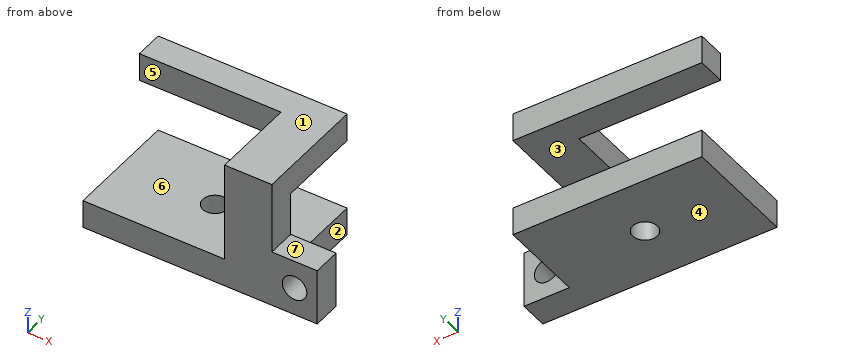
from build123d import *

# Parameters (mm, degrees)
SKETCH1_W               = 100
SKETCH1_H               = 60
BOSS_EXTRUDE1_DEPTH     = 68
SKETCH1_3_W             = 24
SKETCH1_3_H             = 15
BOSS_EXTRUDE2_DEPTH     = 30
SKETCH2_R               = 6.5
CUT_EXTRUDE1_DEPTH      = 40
SKETCH3_W               = 38
SKETCH3_H               = 45
CUT_EXTRUDE2_DEPTH      = 113
CUT_EXTRUDE3_DEPTH      = 105.880884817
CUT_EXTRUDE3_DEPTH_BACK = 53
SKETCH4_W               = 75
SKETCH4_H               = 45
SKETCH5_R               = 6.5
CUT_EXTRUDE4_DEPTH      = 38


with BuildPart() as part:
    # Sketch1 → Boss-Extrude1 (new body)
    with BuildSketch(Plane.XY):
        Rectangle(SKETCH1_W, SKETCH1_H)
    extrude(amount=BOSS_EXTRUDE1_DEPTH)

    # Sketch1_3 → Boss-Extrude2 (add)
    with BuildSketch(Plane.XY):
        with Locations((62, -22.5)):
            Rectangle(SKETCH1_3_W, SKETCH1_3_H)
    extrude(amount=BOSS_EXTRUDE2_DEPTH)

    # Sketch2 → Cut-Extrude1 (cut)
    with BuildSketch(Plane(origin=(0, -15, 0), x_dir=(1, 0, 0), z_dir=(0, 1, 0))):
        with Locations(Location((62, -15, 0), (0, 0, 270))):
            Circle(SKETCH2_R)
    extrude(amount=-CUT_EXTRUDE1_DEPTH, mode=Mode.SUBTRACT)

    # Sketch3 → Cut-Extrude2 (cut)
    with BuildSketch(Plane(origin=(50, 0, 0), x_dir=(0, 0, -1), z_dir=(1, 0, 0))):
        with Locations((-34, 7.5)):
            Rectangle(SKETCH3_W, SKETCH3_H)
    extrude(amount=-CUT_EXTRUDE2_DEPTH, mode=Mode.SUBTRACT)

    # Sketch4 → Cut-Extrude3 (cut, two sides: drawn at the far end of the back side and taken through both)
    with BuildSketch(Plane.XY.offset(68).offset(-CUT_EXTRUDE3_DEPTH_BACK)):
        with Locations((-12.5, -7.5)):
            Rectangle(SKETCH4_W, SKETCH4_H)
    extrude(amount=CUT_EXTRUDE3_DEPTH + CUT_EXTRUDE3_DEPTH_BACK, mode=Mode.SUBTRACT)

    # Sketch5 → Cut-Extrude4 (cut)
    with BuildSketch(Plane(origin=(0, 0, 0), x_dir=(-1, 0, 0), z_dir=(0, 0, -1))):
        Circle(SKETCH5_R)
    extrude(amount=-CUT_EXTRUDE4_DEPTH, mode=Mode.SUBTRACT)


solid = part.part
Verification items for the finished model (mm, model axes). Face numbers are marked on the shaded views. A direction names the side the tool comes from. Round coordinates to 2 decimals unless told otherwise and drop trailing zeros. Loops run counter-clockwise (first coordinate to the right, second up) from the corner with the lowest first, then second, coordinate; pieces in that order, holes last. Notation, with made-up numbers: (41.5, -8) - (59.5, -8) arc R25 cw to (59.5, 20) - close; hole circle Ø3 at (32, 20). An arc over 180 degrees is marked (long way). Use a Markdown table: item, result. Add a question column.
1. Access from +Z, -Z, +X, -X, +Y, -Y to the whole of each face (thin tool, end or side, straight path). Record for the marked faces 5, 6 and 7.
2. Section check C-C, the plane x = 62. Record the boundary of the cut face in (y, z).
3. Release check for a two-part mould opening along Z. For the marked faces 1, 2, 3 and 4 record: released by +Z, released by -Z, zero draft, split by the parting line, or undercut.
4. Section check D-D, the plane y = 8.5. Record the boundary of the cut face in (x, z).
5. Thickness scan on probe 1 along Y at (x, z) = (0, 5); probe 2 along Z at (x, y) = (27, -11); probe 3 along Y at (x, z) = (56.5, 25). Record the ranges inside material, lowest first. Write a range as [from, to].
6. Section check A-A, the plane z = 12.5. Record the boundary of the cut face in (x, y).
7. Section check B-B, the plane x = 0. Record the boundary of the cut face in (y, z), plus the area to 3 significant figures.
8. Gauge pin test, flat ends, axial feed: pin 1 (4 mm diameter, centred on x = 11, y = -18.5, fed in from +Z); pin 2 (4.5 mm diameter, centred on x = -13.5, z = 58, fed in from -Y); pin 3 (7.5 mm diameter, centred on x = 56.5, y = -24, fed in from +Z). Record the tip position at first contact, or that the pin passes through.
Checks:
| question | item | result |
|---|---|---|
| 1 | face 5 | +Z, -X, -Y |
| 1 | face 6 | -X, +Y |
| 1 | face 7 | +Z, +X, +Y, -Y |
| 2 | outline | (-30, 0) - (-15, 0) - (-15, 8.5) - (-30, 8.5) - close; (-30, 21.5) - (-15, 21.5) - (-15, 30) - (-30, 30) - close |
| 3 | face 1 | released by +Z |
| 3 | face 2 | zero draft |
| 3 | face 3 | undercut |
| 3 | face 4 | released by -Z |
| 4 | outline | (-50, 0) - (50, 0) - (50, 15) - (-50, 15) - close; (25, 53) - (50, 53) - (50, 68) - (25, 68) - close |
| 5 | probe 1 | y = [-30, -6.5], [6.5, 30] |
| 5 | probe 2 | z = [0, 15], [53, 68] |
| 5 | probe 3 | y = [-30, -15] |
| 6 | outline | (-50, -30) - (56, -30) - (56, -15) - (50, -15) - (50, 30) - (-50, 30) - close; (68, -30) - (74, -30) - (74, -15) - (68, -15) - close; hole circle Ø13 at (0, 0) |
| 7 | outline | (-30, 0) - (-6.5, 0) - (-6.5, 15) - (-30, 15) - close; (6.5, 0) - (30, 0) - (30, 15) - (6.5, 15) - close; (15, 53) - (30, 53) - (30, 68) - (15, 68) - close |
| 7 | area | 930 mm^2 |
| 8 | pin 1 | stops at z = 15 |
| 8 | pin 2 | stops at y = 15 |
| 8 | pin 3 | stops at z = 30 |
